Verification items for the finished model (mm, model axes). A direction names the side the tool comes from. Coordinates: 2 decimals unless noted, no trailing zeros. Order: outer loops, then holes, each group sorted by start corner. A loop starts at its lowest first (then second) coordinate and runs counter-clockwise, first axis right, second up. Notation, with made-up numbers: M 12,54 L 48,54 A24 ccw 48,90 Z; hole C -20.75,87.5 d11. An arc over 180 degrees is marked long. Use one line per item in the form item = value. Start each with the question number.
```python
from build123d import *

# Parameters (mm, degrees)
F0_W      = 35
F0_H      = 76.5
F1_DEPTH  = 8
F1_FACE_W = 35
F1_FACE_H = 8
F2_W      = 35
F2_H      = 40
F3_DEPTH  = 8
F4_W      = 12.5
F4_H      = 24
F5_DEPTH  = 84.501


with BuildPart() as f1:
    # F0 (on Top) → F1 (new body)
    with BuildSketch(Plane.XY):
        with Locations((0, -38.25)):
            Rectangle(F0_W, F0_H)
    extrude(amount=F1_DEPTH)

    # F1_face (on face) + F2 (on face) → F3 (join)
    with BuildSketch(Plane(origin=(0, -76.5, 4), x_dir=(1, 0, 0), z_dir=(0, -1, 0))):
        Rectangle(F1_FACE_W, F1_FACE_H)
    with BuildSketch(Plane.XZ.offset(76.5)):
        with Locations((0, 20)):
            Rectangle(F2_W, F2_H)
    extrude(amount=F3_DEPTH)

    # F4 (on face) → F5 (cut, through all)
    with BuildSketch(Plane.XZ.offset(84.5)):
        with Locations((0, 20)):
            Rectangle(F4_W, F4_H)
    extrude(amount=-F5_DEPTH, mode=Mode.SUBTRACT)

    # F6: F1 across face


with BuildPart() as f1_1:
    add(f1.part)
    add(f1.part.mirror(Plane(origin=(0, 0, 4), x_dir=(-1, 0, 0), z_dir=(0, 1, 0))))


solid = f1_1.part
```
1. Cross-section at A-A on z = 38.5. Enter the section's corners in (x, y).
2. Release check for a two-part mould opening along X. For faces 1 (the flat face through (-17.5, -19, 7)), 2 (the flat face through (6.25, 81, 20)), 3 (the flat face through (8, -84.5, 20)), 4 (the flat face through (6.25, -81, 20)) record: pulls with the +X half, pulls with the -X half, needs draft (parallel to the pull), parting line crosses it, or undercut.
3. Depth check by flat-ended pin: P1, Ø17.5, axis at x = -8, y = -12, coming from the +Z side. Enter the tip coordinate at first touch or a pass-through.
4. Tool access check on faces 5 (the flat face through (-6.25, -81, 20)), 6 (the flat face through (8, -76.5, 24)), 7 (the flat face through (0, 80, 40)). Record the directions out of +Z, -Z, +X, -X, +Y, -Y that give a thin tool (end or side, any length) a straight path to the whole face; none if there is none.
5. Material ranges on line 1 along Y through (x, z) = (-6.5, 18); line 2 along Z through (x, y) = (-7, -33), recorded low to high.
6. Cross-section at B-B on x = 0. Enter the section's corners in (y, z).
7. Cross-section at D-D on x = -13.5. Enter the section's corners in (y, z), and give its area (3 significant figures).
8. Cross-section at C-C on z = 20.5. Enter the section's corners in (x, y).
Final values:
q1.outline = M -17.5,-84.5 L 17.5,-84.5 L 17.5,-76.5 L -17.5,-76.5 Z; M -17.5,76.5 L 17.5,76.5 L 17.5,84.5 L -17.5,84.5 Z
q2.face_1 = pulls with the -X half
q2.face_2 = undercut
q2.face_3 = needs draft
q2.face_4 = undercut
q3.P1 = 8
q4.face_5 = +Y, -Y
q4.face_6 = +Z, +X, -X
q4.face_7 = +Z, +X, -X, +Y, -Y
q5.line_1 = -84.5 to -76.5, 76.5 to 84.5
q5.line_2 = 0 to 8
q6.outline = M -84.5,0 L 84.5,0 L 84.5,8 L -84.5,8 Z; M -84.5,32 L -76.5,32 L -76.5,40 L -84.5,40 Z; M 76.5,32 L 84.5,32 L 84.5,40 L 76.5,40 Z
q7.outline = M -84.5,0 L 84.5,0 L 84.5,40 L 76.5,40 L 76.5,8 L -76.5,8 L -76.5,40 L -84.5,40 Z
q7.area = 1,860 mm2
q8.outline = M -17.5,-84.5 L -6.25,-84.5 L -6.25,-76.5 L -17.5,-76.5 Z; M -17.5,76.5 L -6.25,76.5 L -6.25,84.5 L -17.5,84.5 Z; M 6.25,-84.5 L 17.5,-84.5 L 17.5,-76.5 L 6.25,-76.5 Z; M 6.25,76.5 L 17.5,76.5 L 17.5,84.5 L 6.25,84.5 Z
